from build123d import *

# Parameters (mm, degrees)
CYLINDER_R      = 20
CYLINDER_DEPTH  = 3.3
SKETCH_R        = 1.5
POCKET_DEPTH    = 3.301
POCKET001_DEPTH = 5


with BuildPart() as part:
    # Cylinder → Cylinder (new body)
    with BuildSketch(Plane.XY):
        Circle(CYLINDER_R)
    extrude(amount=CYLINDER_DEPTH)

    # Sketch (on Face2 of Cylinder) → Pocket (cut, through all)
    with BuildSketch(Plane.XY.offset(3.3)):
        with Locations((0, 15.1)):
            Circle(SKETCH_R)
    extrude(amount=-POCKET_DEPTH, mode=Mode.SUBTRACT)

    # Sketch001 (on Face2 of Pocket) → Pocket001 (cut)
    with BuildSketch(Plane.XY.offset(3.3)):
        Polygon((0.318612, 10.995385), (-8.758163, -6.655418), (8.758163, -6.655418), align=None)
    extrude(amount=-POCKET001_DEPTH, mode=Mode.SUBTRACT)


solid = part.part
Could you check a few things on this model? Use its own coordinates, in mm. A direction names the side the tool comes from. Coordinates: 2 decimals unless noted, no trailing zeros. Order: outer loops, then holes, each group sorted by start corner. A loop starts at its lowest first (then second) coordinate and runs counter-clockwise, first axis right, second up.
Q1. Please list where these lines run through material, in increasing order: L1, parallel to Y at x = 0, z = 2.25; L2, parallel to Y at x = 0.5, z = 2.8; L3, parallel to X at y = -1, z = 1.95.
Q2. Which directions (+Z, -Z, +X, -X, +Y, -Y) give clear straight access to the entire face, cutting with the end or side of a thin tool? Please do faces 4 (the flat face through (4, 5, 0)), 5 (the flat face through (0, -6.655, 2)).
Q3. Suppose I cut it at D-D on x = 13. Please give me the cut outline in (y, z), and give its area (3 significant figures).
Q4. Thinking about a two-plate mould opening in Y: for faces 1 (the flat face through (-4.16, 2.29, 1.67)), 2 (the flat face through (4, 5, 3.3)), 3 (the cylindrical face through (-4.336, -19.524, 1.627)), which applies, released by +Y, released by -Y, zero draft, split by the parting line, or undercut?
Q5. Suppose I cut it at C-C on z = 0.7. Please give me the cut outline in (x, y).
Q6. Will these pins go through, and if not, where does the flat tip stop? pin 1 (4 mm diameter, centred on x = 0, y = 15.1, fed in from -Z); pin 2 (1 mm diameter, centred on x = -15.5, z = 1, fed in from -Y).
Q7. Suppose I cut it at B-B on y = 0. Please give me the cut outline in (x, z).
Q8. Suppose I cut it at A-A on x = 4.5. Please give me the cut outline in (y, z).
Answer:
1. L1: y = -20 to -6.66, 10.38 to 13.6, 16.6 to 20
1. L2: y = -19.99 to -6.66, 10.62 to 13.69, 16.51 to 19.99
1. L3: x = -19.97 to -5.85, 6.05 to 19.97
2. face 4: -Z, +X, -X, +Y, -Y
2. face 5: +Z, -Z
3. outline: (-15.2, 0) - (15.2, 0) - (15.2, 3.3) - (-15.2, 3.3) - close
3. area: 100 mm2
4. face 1: undercut
4. face 2: zero draft
4. face 3: split by the parting line
5. outline: circle Ø40 at (0, 0); hole (-8.76, -6.66) - (8.76, -6.66) - (0.32, 11) - close; hole circle Ø3 at (0, 15.1)
6. pin 1: stops at z = 0
6. pin 2: stops at y = -13.23
7. outline: (-20, 0) - (-5.34, 0) - (-5.34, 3.3) - (-20, 3.3) - close; (5.58, 0) - (20, 0) - (20, 3.3) - (5.58, 3.3) - close
8. outline: (-19.49, 0) - (-6.66, 0) - (-6.66, 3.3) - (-19.49, 3.3) - close; (2.25, 0) - (19.49, 0) - (19.49, 3.3) - (2.25, 3.3) - close
